```python
from build123d import *

# Parameters (mm, degrees)
F1_DEPTH = 20
F4_DEPTH = 20
F2_W     = 2
F2_H     = 20
F5_DEPTH = 12.8
F2_R     = 1.1
F6_DEPTH = 5
F7_W     = 3
F7_H     = 1.5
F7_R     = 1.1
F8_DEPTH = 5
F10_D    = 2.2


with BuildPart() as f1:
    # F0 (on Top) → F1 (new body)
    with BuildSketch(Plane.XY):
        with BuildLine():
            Line((-8.9, -3), (-8.9, 0))
            Line((-8.9, 0), (-12, 0))
            ThreePointArc((-12, 0), (-11.9043563552, -1.5120515098), (-11.6189500386, -3))
            Line((-11.6189500386, -3), (-8.9, -3))
        make_face()
        with BuildLine():
            ThreePointArc((8.9, 0), (0, -8.9), (-8.9, 0))
            Line((-8.9, 0), (-8.9, -3))
            Line((-8.9, -3), (-11.6189500386, -3))
            ThreePointArc((-11.6189500386, -3), (0, -12), (11.6189500386, -3))
            Line((11.6189500386, -3), (8.9, -3))
            Line((8.9, -3), (8.9, 0))
        make_face()
        with BuildLine():
            Line((12, 0), (8.9, 0))
            Line((8.9, 0), (8.9, -3))
            Line((8.9, -3), (11.6189500386, -3))
            ThreePointArc((11.6189500386, -3), (11.9043563552, -1.5120515098), (12, 0))
        make_face()
        with BuildLine():
            ThreePointArc((-11.6189500386, -3), (-11.9043563552, -1.5120515098), (-12, 0))
            Line((-12, 0), (-21.7, 0))
            Line((-21.7, 0), (-21.7, -3))
            Line((-21.7, -3), (-11.6189500386, -3))
        make_face()
        with BuildLine():
            Line((21.7, 0), (12, 0))
            ThreePointArc((12, 0), (11.9043563552, -1.5120515098), (11.6189500386, -3))
            Line((11.6189500386, -3), (21.7, -3))
            Line((21.7, -3), (21.7, 0))
        make_face()
    extrude(amount=-F1_DEPTH)



with BuildPart() as f4:
    # F3 (on Top) → F4 (new body)
    with BuildSketch(Plane.XY):
        with BuildLine():
            Line((-21.7, 2), (-12, 2))
            ThreePointArc((-12, 2), (-11.7273581741, 3.5236938591), (-11.2620660942, 5))
            Line((-11.2620660942, 5), (-21.7, 5))
            Line((-21.7, 5), (-21.7, 2))
        make_face()
        with BuildLine():
            Line((-12, 2), (-8.9, 2))
            Line((-8.9, 2), (-8.9, 5))
            Line((-8.9, 5), (-11.2620660942, 5))
            ThreePointArc((-11.2620660942, 5), (-11.7273581741, 3.5236938591), (-12, 2))
        make_face()
        with BuildLine():
            ThreePointArc((-8.9, 2), (0, 9.662091184), (8.9, 2))
            Line((8.9, 2), (8.9, 5))
            Line((8.9, 5), (11.2620660942, 5))
            ThreePointArc((11.2620660942, 5), (0, 12.7159530528), (-11.2620660942, 5))
            Line((-11.2620660942, 5), (-8.9, 5))
            Line((-8.9, 5), (-8.9, 2))
        make_face()
        with BuildLine():
            ThreePointArc((11.2620660942, 5), (11.7273581741, 3.5236938591), (12, 2))
            Line((12, 2), (21.7, 2))
            Line((21.7, 2), (21.7, 5))
            Line((21.7, 5), (11.2620660942, 5))
        make_face()
        with BuildLine():
            Line((8.9, 5), (8.9, 2))
            Line((8.9, 2), (12, 2))
            ThreePointArc((12, 2), (11.7273581741, 3.5236938591), (11.2620660942, 5))
            Line((11.2620660942, 5), (8.9, 5))
        make_face()
    extrude(amount=-F4_DEPTH)


with BuildPart() as f1_1:
    add(f1.part)

    add(f4.part)  # F5 merges F4
    # F2 (on face) → F5 (join)
    with BuildSketch(Plane.YZ.offset(21.7)):
        with Locations((1, -10)):
            Rectangle(F2_W, F2_H)
    extrude(amount=-F5_DEPTH)

    # F2 (on face) → F6 (join)
    with BuildSketch(Plane.YZ.offset(21.7)):
        Polygon((2, -20), (0, -20), (-3, -20), (-3, -28), (5, -28), (5, -20), align=None)
        with Locations((1, -24)):
            Circle(F2_R, mode=Mode.SUBTRACT)
    extrude(amount=-F6_DEPTH)

    # F7 (on face) → F8 (join)
    with BuildSketch(Plane(origin=(-21.7, 0, 0), x_dir=(0, -1, 0), z_dir=(-1, 0, 0))):
        with Locations((1.5, -20.75)):
            Rectangle(F7_W, F7_H)
        Polygon((3, -28), (3, -21.5), (0, -21.5), (-5, -21.5), (-5, -28), align=None)
        with Locations((-1, -24)):
            Circle(F7_R, mode=Mode.SUBTRACT)
    extrude(amount=-F8_DEPTH)

    # F10 (through all)
    with Locations(Plane(origin=(0, 5, 0), x_dir=(-1, 0, 0), z_dir=(0, 1, 0))):
        with Locations((16.481, -10)):
            Hole(F10_D / 2)


solid = f1_1.part
```
Source: CAD feature listing. Evaluate the final solid. Frame: model axes, mm. A direction names the side the tool comes from. Coordinates: 2 decimals unless noted, no trailing zeros. Write each loop counter-clockwise with the first axis right and the second up, starting at its lowest first coordinate (ties: lowest second). Pieces come first, ordered by that corner, then holes. Notation, with made-up numbers: M 43.5,59 L 87.5,59 A15 ccw 87.5,88 Z; hole C 29,49.5 d6. An arc over 180 degrees is marked long. Answer as a JSON object with one key per item and string values.
1. Cut plane A-A on z = -20.5. Output: boundary loops of the cut face in (x, y), plus the area to 3 significant figures.
Evaluation:
{"outline": "M -21.7,-3 L -16.7,-3 L -16.7,0 L -21.7,0 Z; M 16.7,-3 L 21.7,-3 L 21.7,5 L 16.7,5 Z", "area": "55.0 mm^2"}
2. Contact query for flat-ended pins moving along their axis: P1, Ø6, axis at x = -8, y = -6.5, coming from the -Z side; P2, Ø3, axis at x = -18.5, z = -7, coming from the +Y side; P3, Ø11, axis at x = 14.5, z = -12, coming from the -Y side. Output: stop coordinate, or through.
Evaluation:
{"P1": "z = -20", "P2": "y = 5", "P3": "y = -7.94"}
3. Cut plane D-D on y = 1. Output: boundary loops of the cut face in (x, z), plus the area to 4 significant figures.
Evaluation:
{"outline": "M -21.7,-28 L -16.7,-28 L -16.7,-25.1 L -21.7,-25.1 Z; M -21.7,-22.9 L -16.7,-22.9 L -16.7,-21.5 L -21.7,-21.5 Z; M 8.9,-20 L 16.7,-20 L 16.7,-22.9 L 21.7,-22.9 L 21.7,0 L 8.9,0 Z; M 16.7,-28 L 21.7,-28 L 21.7,-25.1 L 16.7,-25.1 Z", "area": "306.5 mm^2"}
4. Draft query along Y for faces 6 (the cylindrical face through (-0.18, 9.66, -9.86)), 7 (the cylindrical face through (-19.235, 1.238, -25.074)), 8 (the flat face through (-19, 2, -21.5)), 9 (the cylindrical face through (0, -12, -10)). Return one class per face: released by +Y, released by -Y, zero draft, split by the parting line, or undercut.
Evaluation:
{"face 6": "undercut", "face 7": "undercut", "face 8": "zero draft", "face 9": "released by -Y"}
5. Ray query, L1, parallel to X at y = 2.5, z = -22; L2, parallel to Z at x = 17.7, y = 1; L3, parallel to Z at x = -17.85, y = 1. Return the intervals inside material, ascending.
Evaluation:
{"L1": "-21.7 to -16.7, 16.7 to 21.7", "L2": "-28 to -25.1, -22.9 to 0", "L3": "-28 to -25.1, -22.9 to -21.5"}
6. Cut plane B-B on z = -24. Output: boundary loops of the cut face in (x, y).
Evaluation:
{"outline": "M -21.7,-3 L -16.7,-3 L -16.7,-0.1 L -21.7,-0.1 Z; M -21.7,2.1 L -16.7,2.1 L -16.7,5 L -21.7,5 Z; M 16.7,-3 L 21.7,-3 L 21.7,-0.1 L 16.7,-0.1 Z; M 16.7,2.1 L 21.7,2.1 L 21.7,5 L 16.7,5 Z"}
7. Access query for faces 1 (the flat face through (-18, -3, -11)), 2 (the flat face through (17, 5, -11)), 3 (the flat face through (-19, 5, -25)), 4 (the flat face through (-15, 5, -10)), 5 (the flat face through (16.7, 0, -25)). Directions: +Z, -Z, +X, -X, +Y, -Y. A direction counts if a zero-diameter tool reaches every point of the face in a straight line with its end or side. Return the directions, or none.
Evaluation:
{"face 1": "+Z, -Z, -X, -Y", "face 2": "+Z, -Z, +X, +Y", "face 3": "+Z, -Z, +X, -X, +Y", "face 4": "+Z, -Z, -X, +Y", "face 5": "-Z, +Y, -Y"}
8. Cut plane C-C on x = 0. Output: boundary loops of the cut face in (y, z).
Evaluation:
{"outline": "M -12,-20 L -8.9,-20 L -8.9,0 L -12,0 Z; M 9.66,-20 L 12.72,-20 L 12.72,0 L 9.66,0 Z"}
